Input: part model. Units: mm. Frame: model coordinates. Face numbers are marked on the shaded views. Coordinates: 2 decimals unless noted, no trailing zeros. Order: outer loops, then holes, each group sorted by start corner. A loop starts at its lowest first (then second) coordinate and runs counter-clockwise, first axis right, second up. Notation, with made-up numbers: (0, 30) -> (56, 30) arc R17 ccw to (56, 43) -> close; hole circle Ø2 at (44, 71.25). An arc over 180 degrees is marked (long way). Answer as CSV lines item,"result".
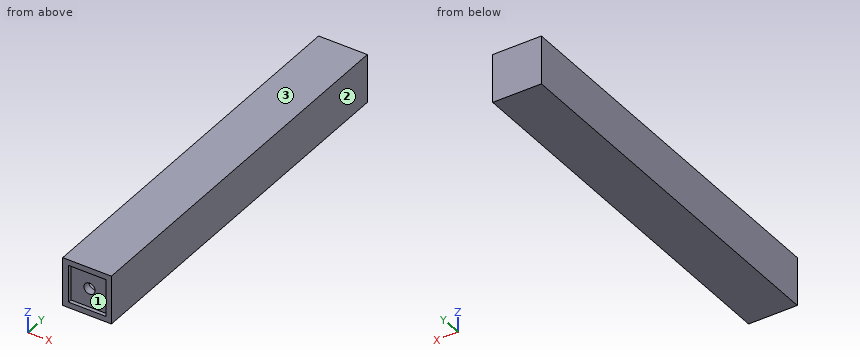
Autodesk Inventor part; units mm, degrees
ref_plane "YZ Plane" through (0, 0, 0) normal (1, 0, 0) x (0, 1, 0)
ref_plane "XZ Plane" through (0, 0, 0) normal (0, 1, 0) x (-1, 0, 0)
ref_plane "XY Plane" through (0, 0, 0) normal (0, 0, 1) x (1, 0, 0)
sketch "Sketch1" plane through (0, 0, 0) normal (0, 1, 0) x (-1, 0, 0)
  circle A0 centre (2.2281, 5.8523) radius 1.5
  circle A1 centre (2.2281, 5.8523) radius 3.5
  line L0 (2.2281, 2.3523) -> (-0.803, 4.1023)
  line L1 (-0.803, 4.1023) -> (-0.803, 7.6023)
  line L2 (-0.803, 7.6023) -> (2.2281, 9.3523)
  line L3 (2.2281, 9.3523) -> (5.2592, 7.6023)
  line L4 (5.2592, 7.6023) -> (5.2592, 4.1023)
  line L5 (5.2592, 4.1023) -> (2.2281, 2.3523)
  point P0 (0, 0)
  dimension "d0" = 7
extrude "Extrusion1" add sketch "Sketch1" against normal blind 2 contours L4 L5 L0 L1 L2 L3
thread "Thread1"
sketch "Sketch2" plane through (0, -2, 0) normal (0, -1, 0) x (1, 0, 0)
  line L0 (-5.2592, 7.6023) -> (-5.2592, 4.1023)
  line L1 (-5.2592, 4.1023) -> (-2.2281, 2.3523)
  line L2 (-2.2281, 2.3523) -> (0.803, 4.1023)
  line L3 (0.803, 4.1023) -> (0.803, 7.6023)
  line L4 (0.803, 7.6023) -> (-2.2281, 9.3523)
  line L5 (-2.2281, 9.3523) -> (-5.2592, 7.6023)
  circle A0 centre (-2.2281, 5.8523) radius 1.5
  line L6 (-7.2281, 0.8523) -> (2.7719, 0.8523)
  line L7 (2.7719, 0.8523) -> (2.7719, 10.8523)
  line L8 (2.7719, 10.8523) -> (-7.2281, 10.8523)
  line L9 (-7.2281, 10.8523) -> (-7.2281, 0.8523)
  line L10 (-7.2281, 0.8523) -> (2.7719, 10.8523) construction
  line L11 (2.7719, 0.8523) -> (-7.2281, 10.8523) construction
  point P0 (0, 0)
  dimension "d5" = 10
  dimension "d6" = 10
extrude "Extrusion2" add sketch "Sketch2" against normal blind 2 contours L9 L8 L7 L6
sketch "Sketch3" plane through (0, 0, 0) normal (0, 1, 0) x (1, 0, 0)
  line L0 (2.7719, -10.8523) -> (2.7719, -0.8523)
  line L1 (2.7719, -0.8523) -> (-7.2281, -0.8523)
  line L2 (-7.2281, -0.8523) -> (-7.2281, -10.8523)
  line L3 (-7.2281, -10.8523) -> (2.7719, -10.8523)
  circle A0 centre (-2.2281, -5.8523) radius 1.5
  line L4 (-8.7281, 0.6477) -> (4.2719, 0.6477)
  line L5 (4.2719, 0.6477) -> (4.2719, -12.3523)
  line L6 (4.2719, -12.3523) -> (-8.7281, -12.3523)
  line L7 (-8.7281, -12.3523) -> (-8.7281, 0.6477)
  line L8 (-8.7281, 0.6477) -> (4.2719, -12.3523) construction
  line L9 (4.2719, 0.6477) -> (-8.7281, -12.3523) construction
  point P0 (0, 0)
  dimension "d9" = 10
  dimension "d10" = 13
  dimension "d11" = 13
extrude "Extrusion3" add sketch "Sketch3" along normal blind 100 and the other way blind 3 contours L4 L5 L6 L7
sketch "Sketch4" plane through (0, 100, 0) normal (0, 1, 0) x (1, 0, 0)
  line L0 (-8.7281, -12.3523) -> (4.2719, -12.3523)
  line L1 (4.2719, -12.3523) -> (4.2719, 0.6477)
  line L2 (4.2719, 0.6477) -> (-8.7281, 0.6477)
  line L3 (-8.7281, 0.6477) -> (-8.7281, -12.3523)
  line L4 (2.7719, -10.8523) -> (-7.2281, -10.8523)
  line L5 (-7.2281, -10.8523) -> (-7.2281, -0.8523)
  line L6 (-7.2281, -0.8523) -> (2.7719, -0.8523)
  line L7 (2.7719, -0.8523) -> (2.7719, -10.8523)
  point P0 (0, 0)
extrude "Extrusion4" add sketch "Sketch4" against normal blind 3 contours L4 L5 L6 L7
properties part number "Nut"
1. Contact query for a flat-ended pin moving along its axis: pin 1 (1.8 mm diameter, centred on x = -2.23, z = 5.85, fed in from -Y). Output: stop coordinate, or through.
Findings:
pin 1,"stops at y = 97"
2. Cut plane B-B (z = 3.5). Return the cut outline in (x, y).
Findings:
outline,"(-8.73, -3) -> (-7.23, -3) -> (-7.23, -2) -> (2.77, -2) -> (2.77, -3) -> (4.27, -3) -> (4.27, 100) -> (-8.73, 100) -> close; hole (-7.23, 0) -> (2.77, 0) -> (2.77, 97) -> (-7.23, 97) -> close"
3. Cut plane C-C (x = 1.5). Return the cut outline in (y, z).
Findings:
outline,"(-3, -0.65) -> (100, -0.65) -> (100, 12.35) -> (-3, 12.35) -> (-3, 10.85) -> (-2, 10.85) -> (-2, 0.85) -> (-3, 0.85) -> close; hole (0, 0.85) -> (97, 0.85) -> (97, 10.85) -> (0, 10.85) -> close"
4. Mould query, pull axis X, two halves, no side actions, for the marked faces 1, 2 and 3. Classes: released by +X, released by -X, zero draft, split by the parting line, or undercut.
Findings:
face 1,"undercut"
face 2,"released by +X"
face 3,"zero draft"
5. Cut plane D-D (x = -2.25). Return the cut outline in (y, z), plus the area to 3 significant figures.
Findings:
outline,"(-3, -0.65) -> (100, -0.65) -> (100, 12.35) -> (-3, 12.35) -> (-3, 10.85) -> (-2, 10.85) -> (-2, 7.35) -> (0, 7.35) -> (0, 10.85) -> (97, 10.85) -> (97, 0.85) -> (0, 0.85) -> (0, 4.35) -> (-2, 4.35) -> (-2, 0.85) -> (-3, 0.85) -> close"
area,"353 mm2"
6. Ray query, line 1 along Z through (x, y) = (1.5, 39); line 2 along Y through (x, z) = (-5.25, 8); line 3 along X through (y, z) = (2.5, 10.75). Return the intervals inside material, ascending.
Findings:
line 1,"z = -0.65 to 0.85, 10.85 to 12.35"
line 2,"y = -2 to 0, 97 to 100"
line 3,"x = -8.73 to -7.23, 2.77 to 4.27"
7. Cut plane A-A (y = 56.5). Return the cut outline in (x, z), plus the area to 3 significant figures.
Findings:
outline,"(-8.73, -0.65) -> (4.27, -0.65) -> (4.27, 12.35) -> (-8.73, 12.35) -> close; hole (-7.23, 0.85) -> (2.77, 0.85) -> (2.77, 10.85) -> (-7.23, 10.85) -> close"
area,"69.0 mm2"
